```python
from build123d import *

# Parameters (mm, degrees)
F2_DEPTH  = 0.6
F3_W      = 12
F3_H      = 5
F4_DEPTH  = 1.5
F5_R      = 0.3
F6_DEPTH  = 0.5
F7_R      = 0.3
F8_DEPTH  = 0.5
F9_R      = 0.75
F10_DEPTH = 0.6
F11_R     = 0.5


with BuildPart() as f2:
    # F1 (on face) → F2 (new body)
    with BuildSketch(Plane.XY):
        Polygon((7, 7), (-18.6, 7), (-18.6, 6.05), (-18.6, -6.05), (-18.6, -7), (7, -7), align=None)
    extrude(amount=F2_DEPTH)

    # F3 (on face) → F4 (join)
    with BuildSketch(Plane.XY.offset(0.6)):
        Polygon((7, 7), (-18.6, 7), (-18.6, 6.05), (-18.6, -6.05), (-18.6, -7), (7, -7), align=None)
        Rectangle(F3_W, F3_H, mode=Mode.SUBTRACT)
    extrude(amount=F4_DEPTH)

    # F5 (on face) → F6 (join)
    with BuildSketch(Plane.XY.offset(2.1)):
        Polygon((7, 7), (-18.6, 7), (-18.6, 6.05), (-18.6, -6.05), (-18.6, -7), (7, -7), align=None)
        with Locations((-5.7, -2.2)):
            Circle(F5_R, mode=Mode.SUBTRACT)
        with Locations((5.7, 2.2)):
            Circle(F5_R, mode=Mode.SUBTRACT)
    extrude(amount=F6_DEPTH)

    # F7 (on face) → F8 (join)
    with BuildSketch(Plane.XY.offset(2.6)):
        Polygon((7, 7), (-18.6, 7), (-18.6, 6.05), (-18.6, -6.05), (-18.6, -7), (7, -7), align=None)
        with BuildLine():
            ThreePointArc((-5.7, -1.9), (-5.4878679656, -1.9878679656), (-5.4, -2.2))
            ThreePointArc((-5.4, -2.2), (-5.4878679656, -2.4121320344), (-5.7, -2.5))
            Line((-5.7, -2.5), (-8.8083426132, -2.5))
            ThreePointArc((-8.8083426132, -2.5), (-16.8562430401, 1.3062430401), (-8.05, 0))
            ThreePointArc((-8.05, 0), (-8.1564552894, -0.9730184354), (-8.4707843891, -1.9))
            Line((-8.4707843891, -1.9), (-5.7, -1.9))
        make_face(mode=Mode.SUBTRACT)
        with Locations((5.7, 2.2)):
            Circle(F7_R, mode=Mode.SUBTRACT)
    extrude(amount=F8_DEPTH)

    # F9 (on face) → F10 (join)
    with BuildSketch(Plane.XY.offset(3.1)):
        Polygon((7, 7), (-18.6, 7), (-18.6, 6.05), (-6.5, 6.05), (-6.5, -6.05), (-18.6, -6.05), (-18.6, -7), (7, -7), align=None)
        with Locations((5.7, 2.2)):
            Circle(F9_R, mode=Mode.SUBTRACT)
    extrude(amount=F10_DEPTH)

    # F11
    f11_edges = [f2.edges().sort_by_distance(p)[0] for p in [
        (4.95, 2.2, 3.7),
    ]]
    fillet(f11_edges, radius=F11_R)


solid = f2.part
```
Here's how the part is built. I have some questions about the finished solid (model axes, mm). A direction names the side the tool comes from. Round coordinates to 2 decimals unless told otherwise and drop trailing zeros. Loops run counter-clockwise (first coordinate to the right, second up) from the corner with the lowest first, then second, coordinate; pieces in that order, holes last.
1. Suppose I cut it at A-A, the plane x = -1.25. Please give me the cut outline in (y, z).
Answers:
outline: (-7, 0) - (7, 0) - (7, 3.7) - (-7, 3.7) - close; hole (-2.5, 0.6) - (2.5, 0.6) - (2.5, 2.1) - (-2.5, 2.1) - close
2. Thinking about a two-plate mould opening in Z: for faces 4 (the face through (-18.6, 0, 2)), 5 (the face through (0, -2.5, 1)), 6 (the face through (-6, 0, 0)), which applies, released by +Z, released by -Z, zero draft, split by the parting line, or undercut?
Answers:
face 4: zero draft
face 5: undercut
face 6: released by -Z
3. Will these pins go through, and if not, where does the flat tip stop? pin 1 (3.5 mm diameter, centred on x = -9.5, y = -1.5, fed in from +Z); pin 2 (0.7 mm diameter, centred on y = 2, z = 3.5, fed in from -X).
Answers:
pin 1: stops at z = 3.1
pin 2: stops at x = -6.5
4. Suppose I cut it at D-D, the plane y = -1.25. Please give me the cut outline in (x, z), and give its area (3 significant figures).
Answers:
outline: (-18.6, 0) - (7, 0) - (7, 3.7) - (-6.5, 3.7) - (-6.5, 3.1) - (-8.23, 3.1) - (-8.23, 2.6) - (-16.87, 2.6) - (-16.87, 3.1) - (-18.6, 3.1) - close; hole (-6, 0.6) - (6, 0.6) - (6, 2.1) - (-6, 2.1) - close
area: 65.1 mm2
5. For faces 1 (the face through (-10, 4, 3.1)), 2 (the face through (-6, -7, 2)), 3 (the face through (-6, 0, 1)), which set-ups out of +Z, -Z, +X, -X, +Y, -Y let a thin tool reach every point of the face, with its end or its side?
Answers:
face 1: +Z, -X
face 2: +Z, -Z, +X, -X, -Y
face 3: none
6. If I drill on probe 1 along Y at (x, z) = (5.7, 2.75); probe 2 along Z at (x, y) = (0.5, -1); probe 3 along X at (y, z) = (-2.2, 2.2), over which ranges is the centre line in solid material (lowest first)?
Answers:
probe 1: y = -7 to 1.9, 2.5 to 7
probe 2: z = 0 to 0.6, 2.1 to 3.7
probe 3: x = -18.6 to -6, -5.4 to 7
7. Suppose I cut it at C-C, the plane x = -12.55. Please give me the cut outline in (y, z).
Answers:
outline: (-7, 0) - (7, 0) - (7, 3.7) - (6.05, 3.7) - (6.05, 3.1) - (4.5, 3.1) - (4.5, 2.6) - (-4.5, 2.6) - (-4.5, 3.1) - (-6.05, 3.1) - (-6.05, 3.7) - (-7, 3.7) - close
8. Suppose I cut it at B-B, the plane z = 1.55. Please give me the cut outline in (x, y).
Answers:
outline: (-18.6, -7) - (7, -7) - (7, 7) - (-18.6, 7) - close; hole (-6, -2.5) - (6, -2.5) - (6, 2.5) - (-6, 2.5) - close
